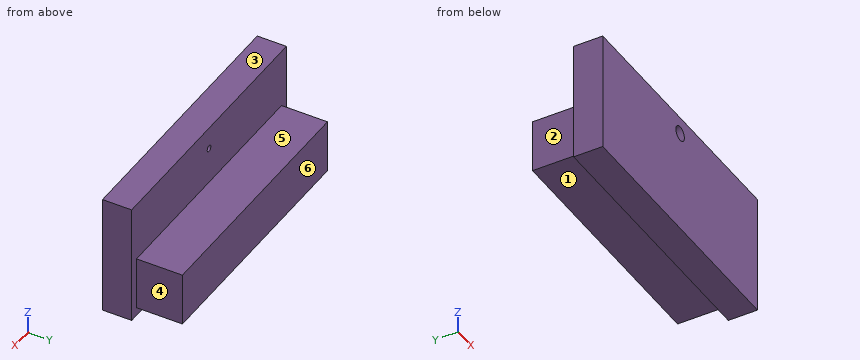
from build123d import *

# Parameters (mm, degrees)
SKETCH1_W           = 120
SKETCH1_H           = 25.630963903
BOSS_EXTRUDE1_DEPTH = 22.019128
SKETCH2_W           = 128
SKETCH2_H           = 58
BOSS_EXTRUDE2_DEPTH = 13.980872
CAVITY1_START       = -22.548845462
CAVITY1_OUTLINE_R   = 3.5
CAVITY1_DEPTH       = 8.988590673
CAVITY1_START_2     = -13.560254789
CAVITY1_2_OUTLINE_R = 1.5
CAVITY1_2_DEPTH     = 6.049448343


# Read off the part's stored shape, not the designer's step: Cavity1
with BuildPart() as part:
    # Sketch1 → Boss-Extrude1 (new body)
    with BuildSketch(Plane.XZ.offset(-14.278818257)):
        with Locations((-20.964398438, -29.724047508)):
            Rectangle(SKETCH1_W, SKETCH1_H)
    extrude(amount=BOSS_EXTRUDE1_DEPTH)


with BuildPart() as boss_extrude2_tool:
    # Sketch2 → Boss-Extrude2 (new body)
    with BuildSketch(Plane.XZ.offset(7.740310225)):
        with Locations((-20.964398438, -17.53952946)):
            Rectangle(SKETCH2_W, SKETCH2_H)
    extrude(amount=BOSS_EXTRUDE2_DEPTH)


with BuildPart() as part_1:
    add(part.part)


with BuildPart() as part_2:
    # Boss-Extrude2: joined with boss_extrude2_tool
    add(part_1.part.fuse(boss_extrude2_tool.part, tol=0.00001))

    # Cavity1 outline → Cavity1 (cut)
    with BuildSketch(Plane(origin=(0, 0, 0), x_dir=(1, 0, 0), z_dir=(0, 0.9857095962326692, -0.16845353037211303)).offset(CAVITY1_START)):
        with Locations((-20.964398438, 0.499578973)):
            Circle(CAVITY1_OUTLINE_R)
    extrude(amount=CAVITY1_DEPTH, mode=Mode.SUBTRACT)

    # Cavity1 2 outline → Cavity1 2 (cut)
    with BuildSketch(Plane(origin=(0, 0, 0), x_dir=(1, 0, 0), z_dir=(0, 0.9857095962326692, -0.16845353037211303)).offset(CAVITY1_START_2)):
        with Locations((-20.964398438, 0.499578973)):
            Circle(CAVITY1_2_OUTLINE_R)
    extrude(amount=CAVITY1_2_DEPTH, mode=Mode.SUBTRACT)


solid = part_2.part
Can you work these out from the model? Positions are in its coordinate system, mm. Face numbers are marked on the shaded views. A direction names the side the tool comes from. Give positions to 0.01 mm unless a question says otherwise; leave off trailing zeros. Loops run counter-clockwise (first coordinate to the right, second up) from the corner with the lowest first, then second, coordinate; pieces in that order, holes last. Notation, with made-up numbers: (19.25, -27.5) -> (24.25, -27.5) arc R15 ccw to (24.25, -20.5) -> close; hole circle Ø5 at (26, -16). An arc over 180 degrees is marked (long way). Write item = value, one per line.
1) Suppose I cut it at A-A on x = -7. Write out the boundary of the cut face in (y, z).
Check result:
outline = (-21.72, -46.54) -> (-7.74, -46.54) -> (-7.74, -42.54) -> (14.28, -42.54) -> (14.28, -16.91) -> (-7.74, -16.91) -> (-7.74, 11.46) -> (-21.72, 11.46) -> close
2) Suppose I cut it at B-B on z = -25. Write out the boundary of the cut face in (x, y).
Check result:
outline = (-84.96, -21.72) -> (43.04, -21.72) -> (43.04, -7.74) -> (39.04, -7.74) -> (39.04, 14.28) -> (-80.96, 14.28) -> (-80.96, -7.74) -> (-84.96, -7.74) -> close
3) Suppose I cut it at D-D on z = -6. Write out the boundary of the cut face in (x, y).
Check result:
outline = (-84.96, -21.72) -> (43.04, -21.72) -> (43.04, -7.74) -> (-84.96, -7.74) -> close
4) Will these pins go through, and if not, where does the flat tip stop? pin 1 (6.5 mm diameter, centred on x = -16.5, y = 5, fed in from +Z); pin 2 (6.5 mm diameter, centred on x = -23.5, y = -2, fed in from -Z); pin 3 (6.5 mm diameter, centred on y = 6, z = -27.5, fed in from +X).
Check result:
pin_1 = -16.91
pin_2 = -42.54
pin_3 = 39.04
5) Suppose I cut it at C-C on y = -2. Write out the boundary of the cut face in (x, z).
Check result:
outline = (-80.96, -42.54) -> (39.04, -42.54) -> (39.04, -16.91) -> (-80.96, -16.91) -> close
6) I need wall thicknesses on L1, parallel to Y at x = -77.5, z = -11; L2, parallel to X at y = -5.5, z = -24.5; L3, parallel to Z at x = 3.5, y = 5. Which ranges of each line are inside material? Lowest first, please. Write a range as from..to.
Check result:
L1 = -21.72..-7.74
L2 = -80.96..39.04
L3 = -42.54..-16.91
7) Thinking about a two-plate mould opening in Z: for the marked faces 1, 2 and 3, which applies, released by +Z, released by -Z, zero draft, split by the parting line, or undercut?
Check result:
face_1 = released by -Z
face_2 = zero draft
face_3 = released by +Z
8) For the marked faces 4, 5 and 6, which set-ups out of +Z, -Z, +X, -X, +Y, -Y let a thin tool reach every point of the face, with its end or its side?
Check result:
face_4 = +Z, -Z, +X, +Y
face_5 = +Z, +X, -X, +Y
face_6 = +Z, -Z, +X, -X, +Y
